Source: CAD feature listing. Evaluate the final solid. Frame: model axes, mm. A direction names the side the tool comes from. Coordinates: 2 decimals unless noted, no trailing zeros. Order: outer loops, then holes, each group sorted by start corner. A loop starts at its lowest first (then second) coordinate and runs counter-clockwise, first axis right, second up. Notation, with made-up numbers: (69, 69) - (121, 69) arc R11 cw to (121, 75) - close; hole circle Ø10 at (21, 78.25). An arc over 180 degrees is marked (long way). One line per question, with ' | ' between items. Start each with the question number.
(1) Section A-A (y = 0). Return the cut outline in (x, z), then the cut area to 3 significant figures.
(2) Section D-D (z = 3.75). Count the separate pieces of the cut face and the enclosed holes in it, then the cut area to 3 significant figures.
(3) Section C-C (y = -14.5). Return the cut outline in (x, z).
(4) Contact query for flat-ended pins moving along their axis: P1, Ø1, axis at y = 17, z = 3, coming from the -X side; P2, Ø1.5, axis at y = 1.5, z = 2.5, coming from the +X side; P3, Ø1.6, axis at y = 28.5, z = 3, coming from the +X side. Output: stop coordinate, or through.
(5) Line query: line 1 along X through (y, z) = (-12, 3.2); line 2 along Y through (x, z) = (-8.5, 4); line 3 along Y through (x, z) = (13, 4.05). Output: solid intervals per line, ascending.
(6) Draft query along X for faces 1 (the flat face through (-1, 1, 4.762)), 2 (the flat face through (-16.4, -16.8, 3.2)), 3 (the cylindrical face through (-11.012, -49.592, 3.153)). Return one class per face: +X half, -X half, draft (parallel to the pull), parting line (faces both ways), or undercut.
(7) Section B-B (x = 0). Return the cut outline in (y, z) (1 decimal), then the cut area to 3 significant figures.
(8) Access query for faces 4 (the flat face through (-1, 1, 1.588)), 5 (the cylindrical face through (-8.27, 4.726, 3.153)). Directions: +Z, -Z, +X, -X, +Y, -Y. A direction counts if a zero-diameter tool reaches every point of the face in a straight line with its end or side. Return the directions, or none.
from build123d import *

# Parameters (mm, degrees)
SKETCH1_R           = 101.6
BOSS_EXTRUDE1_DEPTH = 6.35
SCALE1_SCALE        = 0.5


with BuildPart() as part:
    # Sketch1 → Boss-Extrude1 (new body)
    with BuildSketch(Plane.XY):
        Circle(SKETCH1_R)
        with BuildLine():
            Line((-12.7, 14.199031657), (-12.7, 75.134213245))
            ThreePointArc((-12.7, 75.134213245), (-65.991135768, 38.1), (-71.418137364, -26.568583995))
            Line((-71.418137364, -26.568583995), (-18.646722124, 3.8990068))
            ThreePointArc((-18.646722124, 3.8990068), (-16.497783942, 9.525), (-12.7, 14.199031657))
        make_face(mode=Mode.SUBTRACT)
        with BuildLine():
            Line((12.7, 14.199031657), (12.7, 75.134213245))
            ThreePointArc((12.7, 75.134213245), (65.991135768, 38.1), (71.418137364, -26.568583995))
            Line((71.418137364, -26.568583995), (18.646722124, 3.8990068))
            ThreePointArc((18.646722124, 3.8990068), (16.497783942, 9.525), (12.7, 14.199031657))
        make_face(mode=Mode.SUBTRACT)
        with BuildLine():
            Line((5.946722124, -18.098038457), (58.718137364, -48.565629251))
            ThreePointArc((58.718137364, -48.565629251), (0, -76.2), (-58.718137364, -48.565629251))
            Line((-58.718137364, -48.565629251), (-5.946722124, -18.098038457))
            ThreePointArc((-5.946722124, -18.098038457), (0, -19.05), (5.946722124, -18.098038457))
        make_face(mode=Mode.SUBTRACT)
    extrude(amount=BOSS_EXTRUDE1_DEPTH)


with BuildPart() as part_1:
    # Scale1: scaled about (0, 0, 3.175)
    add(part.part.scale(SCALE1_SCALE).moved(Location((0, 0, 1.5875))))


solid = part_1.part
Response values:
1) outline: (-50.8, 1.59) - (-38.1, 1.59) - (-38.1, 4.76) - (-50.8, 4.76) - close; (-12.7, 1.59) - (12.7, 1.59) - (12.7, 4.76) - (-12.7, 4.76) - close; (38.1, 1.59) - (50.8, 1.59) - (50.8, 4.76) - (38.1, 4.76) - close | area: 161 mm²
2) separate pieces: 1 | enclosed holes: 3 | area: 4,940 mm²
3) outline: (-48.69, 1.59) - (-12.41, 1.59) - (-12.41, 4.76) - (-48.69, 4.76) - close; (12.41, 1.59) - (48.69, 1.59) - (48.69, 4.76) - (12.41, 4.76) - close
4) P1: stops at x = -48.05 | P2: stops at x = 50.79 | P3: stops at x = 42.58
5) line 1: x = -49.36 to -36.16, -33.48 to -8.08, 8.08 to 33.48, 36.16 to 49.36 | line 2: y = -50.08 to -37.14, -12.24 to 4.3, 37.14 to 50.08 | line 3: y = -49.11 to -35.81, -14.84 to -0.17, 35.81 to 49.11
6) face 1: draft | face 2: undercut | face 3: parting line
7) outline: (-50.8, 1.6) - (-38.1, 1.6) - (-38.1, 4.8) - (-50.8, 4.8) - close; (-9.5, 1.6) - (50.8, 1.6) - (50.8, 4.8) - (-9.5, 4.8) - close | area: 232 mm²
8) face 4: -Z, +X, -X, +Y, -Y | face 5: +Z, -Z
